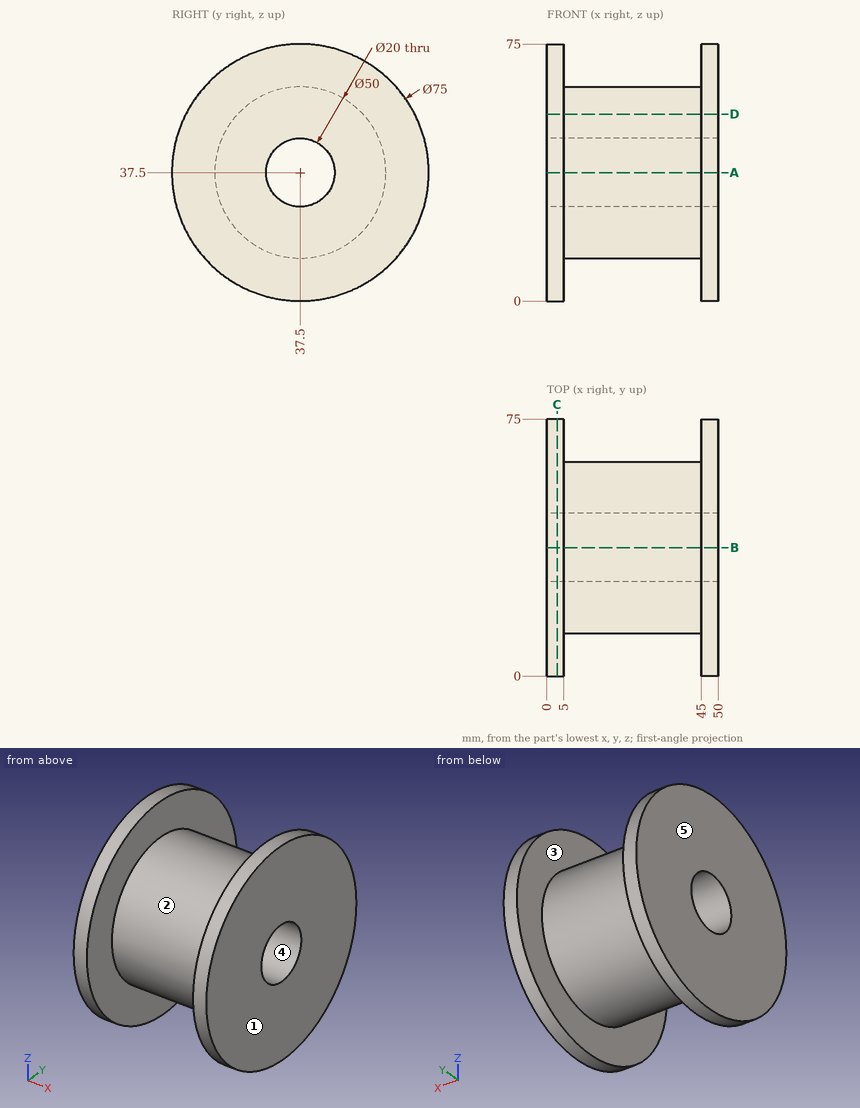
Here's the drawing with two shaded views (mm, measured from the low corner). I have some questions. A direction names the side the tool comes from. Give positions to 0.01 mm unless a question says otherwise; leave off trailing zeros. Loops run counter-clockwise (first coordinate to the right, second up) from the corner with the lowest first, then second, coordinate; pieces in that order, holes last. Notation, with made-up numbers: M -30,-18 L -19,-18 A22 ccw -19,-8 Z; hole C 5,62.25 d10. An arc over 180 degrees is marked long. One line per item, written item: value.
(1) Suppose I cut it at A-A on z = 37.5. List the corners of the cut face in (x, y) for me, plus the area to 3 significant figures.
Returned:
outline: M 0,0 L 5,0 L 5,12.5 L 45,12.5 L 45,0 L 50,0 L 50,27.5 L 0,27.5 Z; M 0,47.5 L 50,47.5 L 50,75 L 45,75 L 45,62.5 L 5,62.5 L 5,75 L 0,75 Z
area: 1,750 mm^2
(2) Suppose I cut it at C-C on x = 3. List the corners of the cut face in (y, z) for me, plus the area to 3 significant figures.
Returned:
outline: C 37.5,37.5 d75; hole C 37.5,37.5 d20
area: 4,100 mm^2
(3) We'd pull the mould along X, two halves only. Please class the marked faces 3, 4 and 5: released by +X, released by -X, zero draft, split by the parting line, or undercut.
Returned:
face 3: undercut
face 4: zero draft
face 5: released by -X
(4) I need wall thicknesses on line 1 (Y direction, x = 25, z = 37) (1 decimal); line 2 (X direction, y = 4, z = 36.5). Which ranges of each line are inside material? Lowest first, please.
Returned:
line 1: 12.5 to 27.5, 47.5 to 62.5
line 2: 0 to 5, 45 to 50
(5) Which directions (+Z, -Z, +X, -X, +Y, -Y) give clear straight access to the entire face, cutting with the end or side of a thin tool? Please do the marked faces 1 and 2.
Returned:
face 1: +Z, -Z, +X, +Y, -Y
face 2: none
(6) Suppose I cut it at D-D on z = 54.5. List the corners of the cut face in (x, y) for me.
Returned:
outline: M 0,4.07 L 5,4.07 L 5,19.17 L 45,19.17 L 45,4.07 L 50,4.07 L 50,70.93 L 45,70.93 L 45,55.83 L 5,55.83 L 5,70.93 L 0,70.93 Z
(7) Will these pins go through, and if not, where does the flat tip stop? pin 1 (2 mm diameter, centred on x = 11.5, z = 58.5, fed in from +Y); pin 2 (10 mm diameter, centred on x = 21, y = 48, fed in from -Z); pin 3 (18 mm diameter, centred on y = 37.5, z = 37.5, fed in from +X); pin 4 (8 mm diameter, centred on x = 34, z = 45.5, fed in from +Y).
Returned:
pin 1: y = 52.5
pin 2: z = 13.11
pin 3: through
pin 4: y = 62.18
